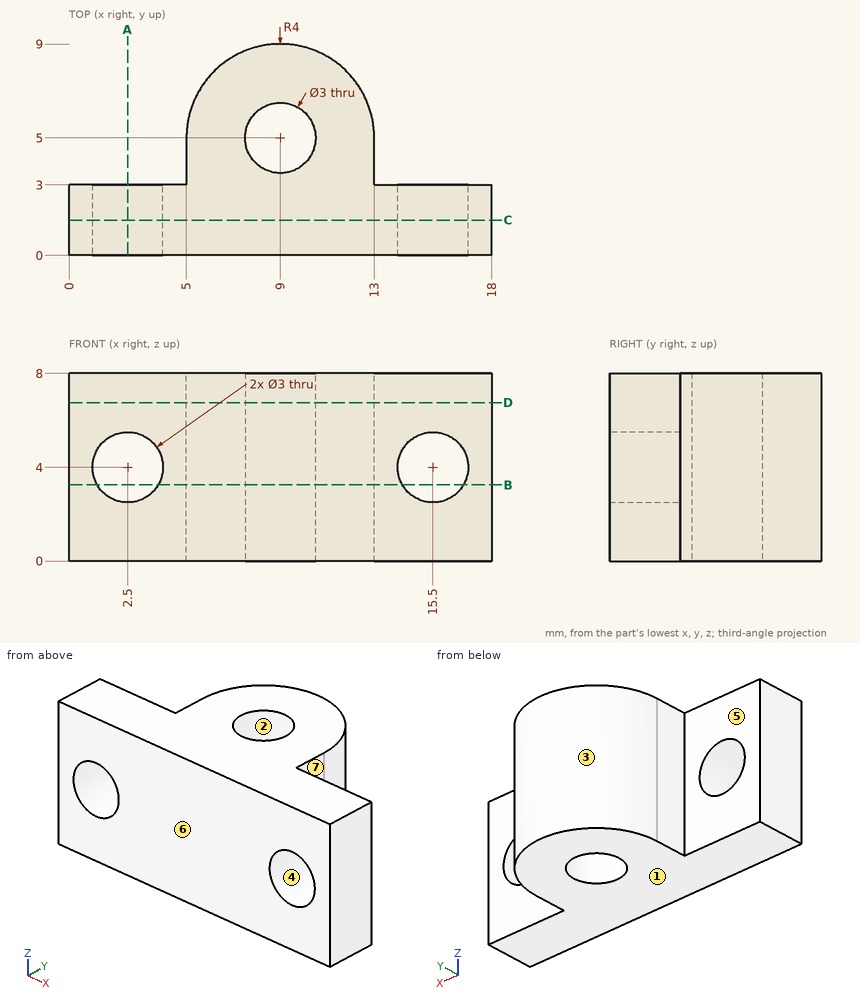
The drawing under review shows one solid part. Ordinate dimensions are in mm from its lowest x, y, z. A direction names the side the tool comes from. Coordinates: 2 decimals unless noted, no trailing zeros. Write each loop counter-clockwise with the first axis right and the second up, starting at its lowest first coordinate (ties: lowest second). Pieces come first, ordered by that corner, then holes. Notation, with made-up numbers: (0, 9) - (49, 9) arc R28 cw to (49, 32) - close; hole circle Ø1 at (65.5, -3). An arc over 180 degrees is marked (long way). Answer in a Markdown table with one row per item. Add a question column.
Q1. For probe 1 along X at (y, z) = (5, 2); probe 2 along Z at (x, y) = (2.5, 0.75); probe 3 along X at (y, z) = (2, 3), list the stretches that pass through material, from the lowest coordinate up.
Q2. Tool access review of the marked faces 5, 6 and 7: name each direction out of +Z, -Z, +X, -X, +Y, -Y from which nothing blocks a thin tool from reaching the whole face with its end or side.
Q3. We need section A-A, the plane x = 2.5. State the section outline as (y, z) points, and give its area (3 significant figures).
Q4. We need section D-D, the plane z = 6.75. State the section outline as (x, y) points, and give its area (3 significant figures).
Q5. Draft analysis for pull direction X (two halves, no side actions). For the marked faces 1, 2, 3 and 4, state which applies: +X half, -X half, draft (parallel to the pull), parting line (faces both ways), or undercut.
Q6. We need section C-C, the plane y = 1.5. State the section outline as (x, z) points.
Q7. We need section B-B, the plane z = 3.25. State the section outline as (x, y) points.
Q8. For P1, Ø2, axis at y = 4.5, z = 3, coming from the -X side; P2, Ø1.5, axis at x = 2, z = 6, coming from the +Y side; P3, Ø2.5, axis at x = 15.5, z = 4, coming from the +Y side; P4, Ø0.6, axis at y = 3.5, z = 4, coming from the +X side, all flat-tipped, find the tip position at first contact; note any pin that passes through.
Answer list:
| question | item | result |
|---|---|---|
| 1 | probe 1 | x = 5 to 7.5, 10.5 to 13 |
| 1 | probe 2 | z = 0 to 2.5, 5.5 to 8 |
| 1 | probe 3 | x = 0 to 1.38, 3.62 to 14.38, 16.62 to 18 |
| 2 | face 5 | +Z, -Z, -X, +Y |
| 2 | face 6 | +Z, -Z, +X, -X, -Y |
| 2 | face 7 | +Z, -Z, +X, +Y |
| 3 | outline | (0, 0) - (3, 0) - (3, 2.5) - (0, 2.5) - close; (0, 5.5) - (3, 5.5) - (3, 8) - (0, 8) - close |
| 3 | area | 15.0 mm2 |
| 4 | outline | (0, 0) - (18, 0) - (18, 3) - (13, 3) - (13, 5) arc R4 ccw to (5, 5) - (5, 3) - (0, 3) - close; hole circle Ø3 at (9, 5) |
| 4 | area | 88.1 mm2 |
| 5 | face 1 | draft |
| 5 | face 2 | undercut |
| 5 | face 3 | parting line |
| 5 | face 4 | undercut |
| 6 | outline | (0, 0) - (18, 0) - (18, 8) - (0, 8) - close; hole circle Ø3 at (2.5, 4); hole circle Ø3 at (15.5, 4) |
| 7 | outline | (0, 0) - (1.2, 0) - (1.2, 3) - (0, 3) - close; (3.8, 0) - (14.2, 0) - (14.2, 3) - (13, 3) - (13, 5) arc R4 ccw to (5, 5) - (5, 3) - (3.8, 3) - close; (16.8, 0) - (18, 0) - (18, 3) - (16.8, 3) - close; hole circle Ø3 at (9, 5) |
| 8 | P1 | stops at x = 5 |
| 8 | P2 | stops at y = 3 |
| 8 | P3 | passes through |
| 8 | P4 | stops at x = 13 |
